Check sheet for the modelled part. Datum: model origin and axes. Units: mm. Give positions to 0.01 mm unless a question says otherwise; leave off trailing zeros. Order: outer loops, then holes, each group sorted by start corner. A loop starts at its lowest first (then second) coordinate and runs counter-clockwise, first axis right, second up. Notation, with made-up numbers: (82.25, 43.25) -> (102.25, 43.25) arc R19 cw to (102.25, 64.25) -> close; hole circle Ø6 at (20, 88.25). An arc over 180 degrees is marked (long way). Write each question's results on one line, items separated by ' | '.
from build123d import *

# Parameters (mm, degrees)
SKETCH1_R           = 2
SKETCH1_R_2         = 2.5
BOSS_EXTRUDE1_DEPTH = 3


with BuildPart() as part:
    # Sketch1 → Boss-Extrude1 (new body)
    with BuildSketch(Plane(origin=(0, 0, 0), x_dir=(0, 0, -1), z_dir=(1, 0, 0))):
        with BuildLine():
            Line((0, 25), (-147, 25))
            ThreePointArc((-147, 25), (-172, 0), (-147, -25))
            Line((-147, -25), (0, -25))
            ThreePointArc((0, -25), (25, 0), (0, 25))
        make_face()
        with BuildLine():
            Line((-132, 20), (-15, 20))
            ThreePointArc((-15, 20), (-25, 0), (-15, -20))
            Line((-15, -20), (-132, -20))
            ThreePointArc((-132, -20), (-122, 0), (-132, 20))
        make_face(mode=Mode.SUBTRACT)
        Circle(SKETCH1_R, mode=Mode.SUBTRACT)
        with Locations((-147, 0)):
            Circle(SKETCH1_R_2, mode=Mode.SUBTRACT)
    extrude(amount=BOSS_EXTRUDE1_DEPTH)


solid = part.part
1. Section check B-B on y = -15. Record the cut outline in (x, z).
Verdict:
outline: (0, -20) -> (3, -20) -> (3, 20) -> (0, 20) -> close; (0, 127) -> (3, 127) -> (3, 167) -> (0, 167) -> close
2. Gauge pin test, flat end, axial feed: pin 1 Ø1.5 at (x, y) = (2, 13) entering from -Z. Record the tip position at first contact, or that the pin passes through.
Verdict:
pin 1: stops at z = -21.79
3. Material ranges on probe 1 along Y at (x, z) = (2.1, 0); probe 2 along Y at (x, z) = (2.85, 45); probe 3 along Z at (x, y) = (2.45, -1), recorded low to high. Write a range as from..to.
Verdict:
probe 1: y = -25..-2, 2..25 | probe 2: y = -25..-20, 20..25 | probe 3: z = -24.98..-1.73, 1.73..24.98, 122.02..144.71, 149.29..171.98
4. Mould release check, pull along Y, two halves, no side actions. Record for faces 1 (the cylindrical face through (1.479, 0.751, 144.615)), 2 (the flat face through (3, -22, 75)), 3 (the cylindrical face through (1.479, 0.55, 171.994)), 4 (the cylindrical face through (1, 0, 25)): +Y half, -Y half, draft (parallel to the pull), parting line (faces both ways), or undercut.
Verdict:
face 1: undercut | face 2: draft | face 3: parting line | face 4: undercut
5. Section check C-C on z = 76. Record the cut outline in (x, y), then the cut area to 3 significant figures.
Verdict:
outline: (0, -25) -> (3, -25) -> (3, -20) -> (0, -20) -> close; (0, 20) -> (3, 20) -> (3, 25) -> (0, 25) -> close | area: 30.0 mm^2
6. Section check A-A on x = 2.05. Record the cut outline in (y, z).
Verdict:
outline: (-25, 0) arc R25 ccw to (25, 0) -> (25, 147) arc R25 ccw to (-25, 147) -> close; hole (-20, 15) arc R25 cw to (20, 15) -> (20, 132) arc R25 cw to (-20, 132) -> close; hole circle Ø5 at (0, 147); hole circle Ø4 at (0, 0)
7. Section check D-D on y = 0. Record the cut outline in (x, z).
Verdict:
outline: (0, -25) -> (3, -25) -> (3, -2) -> (0, -2) -> close; (0, 2) -> (3, 2) -> (3, 25) -> (0, 25) -> close; (0, 122) -> (3, 122) -> (3, 144.5) -> (0, 144.5) -> close; (0, 149.5) -> (3, 149.5) -> (3, 172) -> (0, 172) -> close
